from build123d import *

# Parameters (mm, degrees)
HOLE_WIZARD_M81_D     = 6.8
HOLE_WIZARD_M81_DEPTH = 22.25
HOLE_WIZARD_M81_TIP   = 2.042926105
FILLET_1_R            = 1


with BuildPart() as part:
    # Эскиз1 → Повернуть1 (revolve)
    with BuildSketch(Plane.XY, mode=Mode.PRIVATE) as revolve_1_sk:
        Polygon((0, 0), (0, 20), (52, 20), (52, 25), (121.5, 25), (121.5, 32.5), (129, 32.5), (129, 28.5), (179, 28.5), (179, 0), align=None)
    revolve(revolve_1_sk.sketch.rotate(Axis((0, 0, 0), (1, 0, 0)), 90), axis=Axis((0, 0, 0), (1, 0, 0)))

    # Отверстие обработанное метчиком M81
    with Locations(Plane.ZY):
        with Locations((0, 0)):
            Hole(HOLE_WIZARD_M81_D / 2, depth=HOLE_WIZARD_M81_DEPTH)
            with Locations((0, 0, -(HOLE_WIZARD_M81_DEPTH + HOLE_WIZARD_M81_TIP / 2))):  # 118° drill point
                Cone(0, HOLE_WIZARD_M81_D / 2, HOLE_WIZARD_M81_TIP, mode=Mode.SUBTRACT)

    # Скругление1
    fillet_1_edges = [part.edges().sort_by_distance(p)[0] for p in [
        (52, 0, -25),
        (0, 0, -20),
        (179, 0, -28.5),
        (129, 0, -32.5),
        (121.5, 0, -32.5),
    ]]
    fillet(fillet_1_edges, radius=FILLET_1_R)


solid = part.part
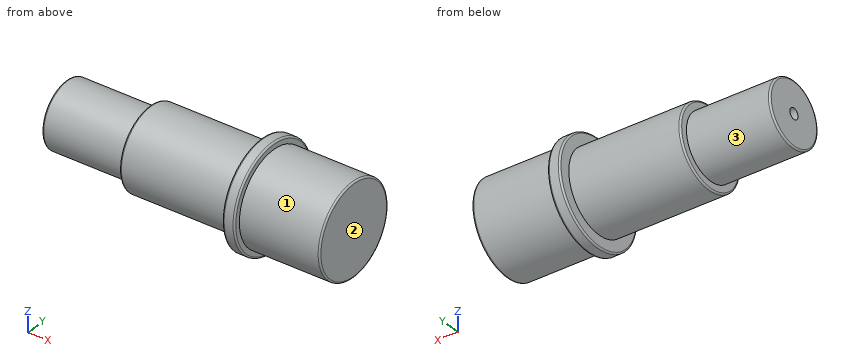
Verification items for the finished model (mm, model axes). Face numbers are marked on the shaded views. A direction names the side the tool comes from. Round coordinates to 2 decimals unless told otherwise and drop trailing zeros. Loops run counter-clockwise (first coordinate to the right, second up) from the corner with the lowest first, then second, coordinate; pieces in that order, holes last. Notation, with made-up numbers: (88.25, -22.5) - (103.25, -22.5) arc R25 ccw to (103.25, -5.5) - close; hole circle Ø2 at (88.5, 52.25). An arc over 180 degrees is marked (long way). Answer in a Markdown table with one row per item. Add a question column.
Q1. Section check A-A on x = 116.5. Enter the section's corners in (y, z).
Q2. Section check B-B on x = 163.5. Enter the section's corners in (y, z), plus the area to 3 significant figures.
Q3. Gauge pin test, flat ends, axial feed: pin 1 (5 mm diameter, centred on x = 130.5, y = 17, fed in from -Z); pin 2 (2 mm diameter, centred on x = 98.5, y = 1, fed in from -Z); pin 3 (3 mm diameter, centred on x = 88.5, y = -5, fed in from +Z). Record the tip position at first contact, or that the pin passes through.
Q4. Tool access check on the marked faces 1, 2 and 3. Record the directions out of +Z, -Z, +X, -X, +Y, -Y that give a thin tool (end or side, any length) a straight path to the whole face; none if there is none.
Q5. Material ranges on line 1 (Y direction, x = 15.25, z = 0); line 2 (X direction, y = -21.5, z = -22); line 3 (X direction, y = -24, z = -7.5), recorded low to high.
Found:
| question | item | result |
|---|---|---|
| 1 | outline | circle Ø50 at (0, 0) |
| 2 | outline | circle Ø57 at (0, 0) |
| 2 | area | 2,550 mm² |
| 3 | pin 1 | stops at z = -28.41 |
| 3 | pin 2 | stops at z = -25 |
| 3 | pin 3 | stops at z = 24.75 |
| 4 | face 1 | +X |
| 4 | face 2 | +Z, -Z, +X, +Y, -Y |
| 4 | face 3 | -X |
| 5 | line 1 | y = -20 to -3.4, 3.4 to 20 |
| 5 | line 2 | x = 121.5 to 129 |
| 5 | line 3 | x = 121.5 to 179 |
